The model under review builds one solid part; all positions refer to its coordinate system, in mm. Face numbers are marked on the shaded views. A direction names the side the tool comes from. Give positions to 0.01 mm unless a question says otherwise; leave off trailing zeros. Loops run counter-clockwise (first coordinate to the right, second up) from the corner with the lowest first, then second, coordinate; pieces in that order, holes last. Notation, with made-up numbers: M 52.25,88 L 67.25,88 A17 cw 67.25,92 Z; hole C 66,12.25 d4. An arc over 180 degrees is marked long. One line per item, written item: value. Start each with the question number.
Q1. For the marked faces 1 and 2, list the 3-axis set-ups (+Z, -Z, +X, -X, +Y, -Y) from which the entire face can be reached by the end or side of a thin tool; tool diameter is ignored.
Q2. To check wall thickness, follow line 1 along Z through (x, y) = (-7.25, -2.9); line 2 along X through (y, z) = (23, 74); line 3 along Y through (x, z) = (-9, 68). State the ranges of each line that lie inside material, in increasing order. Write a range as from..to.
Q3. We need section A-A on x = 8.25. Write out the cut boundary in (y, z).
Q4. For pin 1 (2 mm diameter, centred on x = -18, z = 17, fed in from +Y), flat-tipped, find the tip position at first contact; note if it passes through.
Q5. We need section C-C on y = 12. Write out the cut boundary in (x, z).
Q6. We need section B-B on y = 8. Write out the cut boundary in (x, z).
Q7. Mouldability with a two-part tool opening along X and no side actions: class the marked faces 3, 4 and 5 as released by +X, released by -X, zero draft, split by the parting line, or undercut.
Q8. We need section D-D on x = -15. Write out the cut boundary in (y, z).
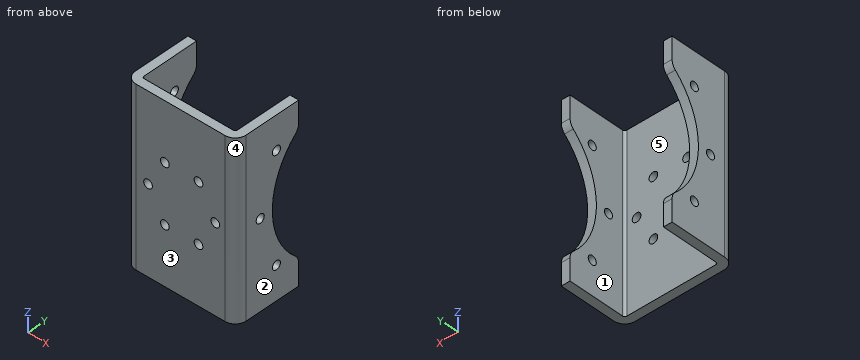
```python
from build123d import *

# Parameters (mm, degrees)
SM_BASE_FLANGE_1_DEPTH   = 80
CUT_EXTRUDE_3_DEPTH      = 99.640762365
CUT_EXTRUDE_3_DEPTH_BACK = 99.640762365
SKETCH_6_R               = 36
SKETCH_6_R_2             = 2
FILLET_1_R               = 5
SKETCH_9_R               = 2
CUT_EXTRUDE_4_DEPTH      = 90.505586418


# Sheet-metal steps are written as plain solids
with BuildPart() as part:
    # Sketch 1 → Базовая кромка1 (new body)
    with BuildSketch(Plane.XY):
        with BuildLine():
            Line((-21.5, 27), (-21.5, 1))
            ThreePointArc((-21.5, 1), (-21.207106781, 0.292893219), (-20.5, 0))
            Line((-20.5, 0), (20.5, 0))
            ThreePointArc((20.5, 0), (21.207106781, 0.292893219), (21.5, 1))
            Line((21.5, 1), (21.5, 27))
            Line((21.5, 27), (25.5, 27))
            Line((25.5, 27), (25.5, 1))
            ThreePointArc((25.5, 1), (24.035533906, -2.535533906), (20.5, -4))
            Line((20.5, -4), (-20.5, -4))
            ThreePointArc((-20.5, -4), (-24.035533906, -2.535533906), (-25.5, 1))
            Line((-25.5, 1), (-25.5, 27))
            Line((-25.5, 27), (-21.5, 27))
        make_face()
    extrude(amount=SM_BASE_FLANGE_1_DEPTH)

    # Эскиз6 → Вырез-Вытянуть3 (cut, two sides: drawn at the far end of the back side and taken through both)
    with BuildSketch(Plane.ZY.offset(25.5).offset(-CUT_EXTRUDE_3_DEPTH_BACK)):
        with Locations((40, 50)):
            Circle(SKETCH_6_R)
        with Locations((40, 8)):
            Circle(SKETCH_6_R_2)
        with Locations((15.313019404, 16.021286236)):
            Circle(SKETCH_6_R_2)
        with Locations((64.686980596, 16.021286236)):
            Circle(SKETCH_6_R_2)
    extrude(amount=CUT_EXTRUDE_3_DEPTH + CUT_EXTRUDE_3_DEPTH_BACK, mode=Mode.SUBTRACT)

    # Скругление1
    fillet_1_edges = [part.edges().sort_by_distance(p)[0] for p in [
        (23.5, 27, 12.305235152),
        (23.5, 27, 67.694764848),
        (-23.5, 27, 12.305235152),
        (-23.5, 27, 67.694764848),
    ]]
    fillet(fillet_1_edges, radius=FILLET_1_R)

    # Эскиз9 → Вырез-Вытянуть4 (cut, through all)
    with BuildSketch(Plane.XZ.offset(4)):
        with Locations((16, 40)):
            Circle(SKETCH_9_R)
        with Locations((8.25, 26.576606241)):
            Circle(SKETCH_9_R)
        with Locations((-7.25, 26.576606241)):
            Circle(SKETCH_9_R)
        with Locations((-15, 40)):
            Circle(SKETCH_9_R)
        with Locations((-7.25, 53.423393759)):
            Circle(SKETCH_9_R)
        with Locations((8.25, 53.423393759)):
            Circle(SKETCH_9_R)
    extrude(amount=-CUT_EXTRUDE_4_DEPTH, mode=Mode.SUBTRACT)


solid = part.part
```
Solved:
1. face 1: +Z, -Z, +Y
1. face 2: +Z, -Z, +X, +Y, -Y
2. line 1: 0..24.58, 28.58..51.42, 55.42..80
2. line 2: -25.5..-21.5, 21.5..25.5
2. line 3: -4..0
3. outline: M -4,0 L 0,0 L 0,24.58 L -4,24.58 Z; M -4,28.58 L 0,28.58 L 0,51.42 L -4,51.42 Z; M -4,55.42 L 0,55.42 L 0,80 L -4,80 Z
4. pin 1: y = 0
5. outline: M -25.5,0 L -21.5,0 L -21.5,80 L -25.5,80 Z; M 21.5,0 L 25.5,0 L 25.5,80 L 21.5,80 Z
6. outline: M -25.5,0 L -21.5,0 L -21.5,38 L -25.5,38 Z; M -25.5,42 L -21.5,42 L -21.5,80 L -25.5,80 Z; M 21.5,0 L 25.5,0 L 25.5,38 L 21.5,38 Z; M 21.5,42 L 25.5,42 L 25.5,80 L 21.5,80 Z
7. face 3: zero draft
7. face 4: released by +X
7. face 5: undercut
8. outline: M -4,0 L 0,0 L 0,38 L -4,38 Z; M -4,42 L 0,42 L 0,80 L -4,80 Z
